```python
from build123d import *
from OCP.BRepFilletAPI import BRepFilletAPI_MakeChamfer

# Parameters (mm, degrees)
SKETCH1_R           = 57.5
BOSS_EXTRUDE1_DEPTH = 600
SKETCH2_R           = 48.722615626
CUT_EXTRUDE1_DEPTH  = 606.485342515
CHAMFER1_SIZE       = 4.866916
CHAMFER1_SIZE2      = 2.809915


with BuildPart() as part:
    # Sketch1 → Boss-Extrude1 (new body)
    with BuildSketch(Plane(origin=(0, 0, 0), x_dir=(1, 0, 0), z_dir=(0, 1, 0))):
        with Locations(Location((0, 0, 0), (0, 0, 270))):
            Circle(SKETCH1_R)
    extrude(amount=BOSS_EXTRUDE1_DEPTH)

    # Sketch2 → Cut-Extrude1 (cut, through all)
    with BuildSketch(Plane(origin=(0, 0, 0), x_dir=(1, 0, 0), z_dir=(0, 1, 0))):
        with Locations(Location((0, 0, 0), (0, 0, 270))):
            Circle(SKETCH2_R)
    extrude(amount=CUT_EXTRUDE1_DEPTH, mode=Mode.SUBTRACT)

    # Chamfer1: one chamfer whose edges measure the first distance from different faces: ONE call of the kernel's chamfer builder (chamfer() names one face for all edges)
    chamfer1_edges_1 = [part.edges().sort_by_distance(p)[0] for p in [
        (0, 0, -57.5),
    ]]
    chamfer1_side_1 = [part.faces().sort_by_distance(p)[0] for p in [
        (0, 0, -55.873654403),
    ]]
    chamfer1_edges_2 = [part.edges().sort_by_distance(p)[0] for p in [
        (0, 600, -57.5),
    ]]
    chamfer1_side_2 = [part.faces().sort_by_distance(p)[0] for p in [
        (0, 300, -57.5),
    ]]
    chamfer1 = BRepFilletAPI_MakeChamfer(part.part.solid().wrapped)
    for e in chamfer1_edges_1:
        chamfer1.Add(CHAMFER1_SIZE, CHAMFER1_SIZE2, e.wrapped, chamfer1_side_1[0].wrapped)  # the first distance lies on this face
    for e in chamfer1_edges_2:
        chamfer1.Add(CHAMFER1_SIZE, CHAMFER1_SIZE2, e.wrapped, chamfer1_side_2[0].wrapped)  # the first distance lies on this face
    add(Compound.cast(chamfer1.Shape()), mode=Mode.REPLACE)


solid = part.part
```
Geometry: final body of the model. Coordinates: model frame, mm. Round coordinates to 2 decimals unless told otherwise and drop trailing zeros. Loops run counter-clockwise (first coordinate to the right, second up) from the corner with the lowest first, then second, coordinate; pieces in that order, holes last. Notation, with made-up numbers: (13, -32) -> (71, -32) arc R32 ccw to (71, 7) -> close; hole circle Ø6 at (-4, 73). An arc over 180 degrees is marked (long way). Use one line per item in the form item = value. Start each with the question number.
1) Section A-A on x = 0. Output: boundary loops of the cut face in (y, z), then the cut area to 3 significant figures.
2) Section C-C on y = 363.5. Output: boundary loops of the cut face in (x, z).
3) Line query: L1, parallel to X at y = 317, z = 0; L2, parallel to Z at x = 12.5, y = 289; L3, parallel to Z at x = 4, y = 223.5. Output: solid intervals per line, ascending.
4) First-contact query: P1, Ø10, axis at y = 444, z = -36.5, coming from the +X side; P2, Ø3, axis at x = 22.5, y = 488.5, coming from the +Z side; P3, Ø1.5, axis at y = 72.5, z = -3, coming from the +X side. Flat tips, straight axial feed; report the tip coordinate or a pass-through.
5) Section B-B on z = 0. Output: boundary loops of the cut face in (x, y).
Response:
q1.outline = (0, -52.63) -> (2.81, -57.5) -> (595.13, -57.5) -> (600, -54.69) -> (600, -48.72) -> (0, -48.72) -> close; (0, 48.72) -> (600, 48.72) -> (600, 54.69) -> (595.13, 57.5) -> (2.81, 57.5) -> (0, 52.63) -> close
q1.area = 10,500 mm^2
q2.outline = circle Ø115 at (0, 0); hole circle Ø97.45 at (0, 0)
q3.L1 = -57.5 to -48.72, 48.72 to 57.5
q3.L2 = -56.12 to -47.09, 47.09 to 56.12
q3.L3 = -57.36 to -48.56, 48.56 to 57.36
q4.P1 = 48.1
q4.P2 = 53.53
q4.P3 = 57.46
q5.outline = (-57.5, 2.81) -> (-52.63, 0) -> (-48.72, 0) -> (-48.72, 600) -> (-54.69, 600) -> (-57.5, 595.13) -> close; (48.72, 0) -> (52.63, 0) -> (57.5, 2.81) -> (57.5, 595.13) -> (54.69, 600) -> (48.72, 600) -> close
